Answer from the drawing. Dimensions are ordinates in mm from the lowest x, y and z of the part. Coordinates: 2 decimals unless noted, no trailing zeros. Order: outer loops, then holes, each group sorted by start corner. A loop starts at its lowest first (then second) coordinate and runs counter-clockwise, first axis right, second up. Notation, with made-up numbers: (-19, -9) - (26, -9) arc R14 ccw to (26, -3) - close; hole circle Ø6 at (-19.5, 57). An arc over 180 degrees is marked (long way). One line per item, written item: value. Start each with the question number.
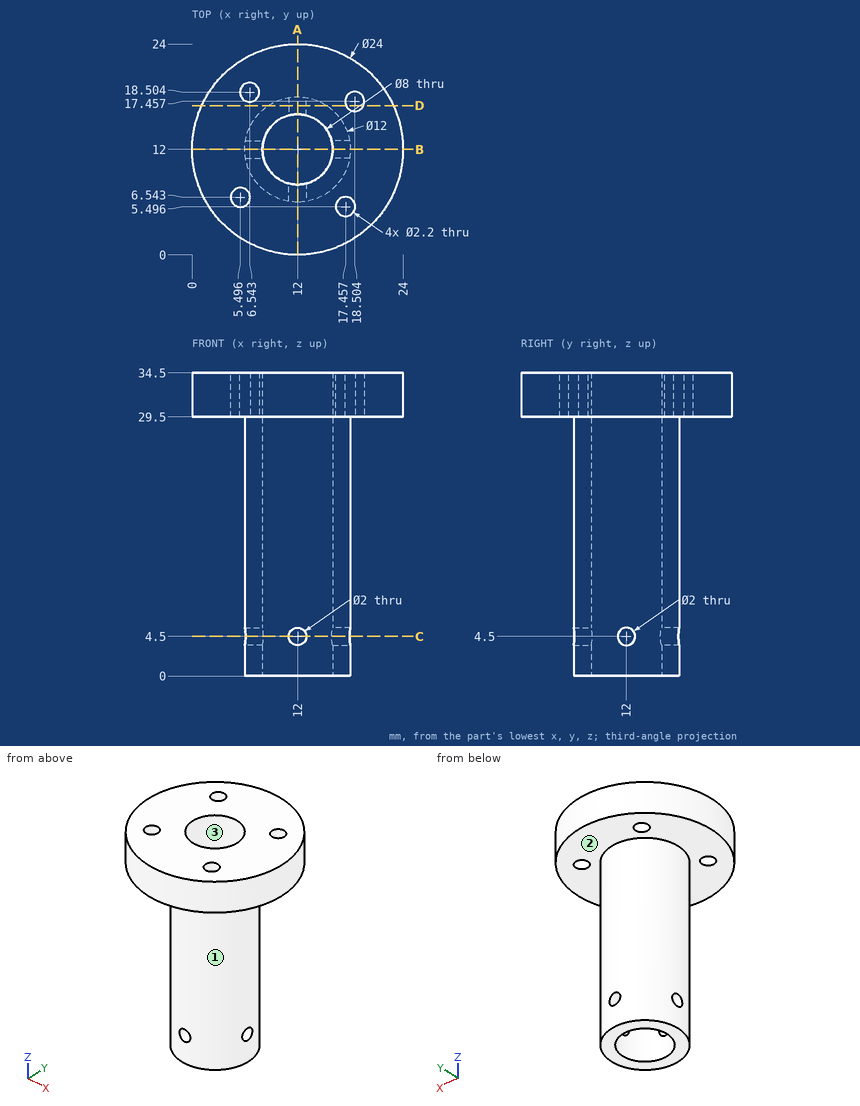
(1) Consider probe 1 along Y at (x, z) = (11.75, 20) (1 decimal); probe 2 along Y at (x, z) = (11.75, 32). Determine where each line is inside the solid, lowest interval first.
(2) The part is cut by section C-C on z = 4.5. Determine the outline of the cut face in (x, y).
(3) The part is cut by section A-A on x = 12. Determine the outline of the cut face in (y, z).
(4) For a pull along X with two mould halves and no side action, classify the marked faces 1, 2 and 3 as pulls with the +X half, pulls with the -X half, needs draft (parallel to the pull), parting line crosses it, or undercut.
(5) The part is cut by section D-D on y = 17. Determine the outline of the cut face in (x, z), plus the area to 3 significant figures.
(6) Flat-ended cylindrical pins translate along their axes: pin 1 Ø8 at (y, z) = (17, 19.5) entering from +X; pin 2 Ø2.5 at (x, z) = (12, 4.5) entering from -Y; pin 3 Ø1.8 at (x, y) = (5.5, 6.54) entering from -Z; pin 4 Ø1.5 at (x, y) = (16.5, 7.5) entering from -Z. Find the tip coordinate at first contact, or state that the pin passes through.
Completed:
1. probe 1: y = 6 to 8, 16 to 18
1. probe 2: y = 0 to 8.01, 15.99 to 24
2. outline: (6.08, 11) arc R6 ccw to (11, 6.08) - (11, 8.13) arc R4 cw to (8.13, 11) - close; (6.08, 13) - (8.13, 13) arc R4 cw to (11, 15.87) - (11, 17.92) arc R6 ccw to start; (13, 6.08) arc R6 ccw to (17.92, 11) - (15.87, 11) arc R4 cw to (13, 8.13) - close; (13, 15.87) arc R4 cw to (15.87, 13) - (17.92, 13) arc R6 ccw to (13, 17.92) - close
3. outline: (0, 29.5) - (6, 29.5) - (6, 5.5) - (8, 5.5) - (8, 34.5) - (0, 34.5) - close; (6, 0) - (8, 0) - (8, 3.5) - (6, 3.5) - close; (16, 0) - (18, 0) - (18, 3.5) - (16, 3.5) - close; (16, 5.5) - (18, 5.5) - (18, 29.5) - (24, 29.5) - (24, 34.5) - (16, 34.5) - close
4. face 1: parting line crosses it
4. face 2: needs draft
4. face 3: undercut
5. outline: (1.09, 29.5) - (8.68, 29.5) - (8.68, 0) - (15.32, 0) - (15.32, 29.5) - (17.5, 29.5) - (17.5, 34.5) - (1.09, 34.5) - close; (19.5, 29.5) - (22.91, 29.5) - (22.91, 34.5) - (19.5, 34.5) - close; hole circle Ø2 at (12, 4.5)
5. area: 292 mm2
6. pin 1: stops at x = 17.92
6. pin 2: stops at y = 6
6. pin 3: passes through
6. pin 4: stops at z = 0
